Work out the finished part from the listing and answer in its coordinate system (mm). A direction names the side the tool comes from. Give positions to 0.01 mm unless a question says otherwise; leave off trailing zeros. Write each loop counter-clockwise with the first axis right and the second up, starting at its lowest first coordinate (ties: lowest second). Pieces come first, ordered by that corner, then holes. Notation, with made-up numbers: (65.25, -9) -> (112.25, -9) arc R6 cw to (112.25, -3) -> close; hole circle Ø2 at (86.5, 66). An arc over 180 degrees is marked (long way). Use a Markdown table: item, result. Add a question column.
Q1. For a pull along Z with two mould halves and no side action, classify faces 1 (the face through (0, 20, -51)), 2 (the face through (172, 39, -100)), 3 (the face through (180, 60, -93.12)), 4 (the face through (323.197, 20.28, -54.391)) as pulls with the +Z half, pulls with the -Z half, needs draft (parallel to the pull), parting line crosses it, or undercut.
Q2. Each of these flat-tipped pins is pushed along its axis until it touches: pin 1 Ø12 at (x, z) = (263, -63.5) entering from +Y; pin 2 Ø2 at (y, z) = (52.5, -96.5) entering from -X; pin 3 Ø5 at (x, y) = (210.5, 40) entering from +Z; pin 4 Ø0.5 at (x, y) = (339, 64) entering from +Z. Where does it stop, or does it pass through?
Q3. Section D-D, the plane z = -59.5 is taken. Give the vertices of the cut face in (x, y), plus the area to 3 significant figures.
Q4. Consider line 1 (X direction, y = 5, z = -65.5); line 2 (X direction, y = 13.5, z = -64.5); line 3 (Y direction, x = 285.5, z = -70). Determine where each line is inside the solid, lowest interval first.
Q5. For faces 5 (the face through (33.144, 60, -97)), 6 (the face through (340, 22, -49)), 7 (the face through (331.968, 60, -46)), 8 (the face through (231, 80, -95)), 9 (the face through (338.282, 60, -47)), determine the directions among +Z, -Z, +X, -X, +Y, -Y from which every point of the face is accessible in a straight line to the end or side of a thin tool.
Q6. Section B-B, the plane x = 82.5 is taken. Give the vertices of the cut face in (y, z).
Q7. Section A-A, the plane z = -12 is taken. Give the vertices of the cut face in (x, y), plus the area to 3 significant figures.
Q8. Section C-C, the plane y = 51 is taken. Give the vertices of the cut face in (x, z).
Autodesk Inventor part; units mm, degrees
ref_plane "YZ Plane" through (0, 0, 0) normal (1, 0, 0) x (0, 1, 0)
ref_plane "XZ Plane" through (0, 0, 0) normal (0, 1, 0) x (-1, 0, 0)
ref_plane "XY Plane" through (0, 0, 0) normal (0, 0, 1) x (1, 0, 0)
sketch "Sketch1" plane through (0, 0, 0) normal (0, 1, 0) x (-1, 0, 0)
  line L0 (0, 0) -> (-340, 0)
  line L1 (-340, 0) -> (-340, -100)
  line L2 (-340, -100) -> (0, -100)
  line L3 (0, -100) -> (0, 0)
  dimension "d0" = 340
  dimension "d1" = 100
extrude "Extrusion1" add sketch "Sketch1" along normal blind 40
sketch "Sketch2" plane through (0, 40, 0) normal (0, 1, 0) x (1, 0, 0)
  circle A0 centre (302.5068, 47.875) radius 21.6916
  circle A1 centre (202.5481, 47.875) radius 21.6916
  circle A2 centre (96.2761, 47.875) radius 21.6916
  circle A3 centre (302.5068, 47.875) radius 21.6916
  point P0 (0, 0)
extrude "Extrusion2" cut sketch "Sketch2" against normal blind 500
sketch "Sketch3" plane through (0, 40, 0) normal (0, 1, 0) x (1, 0, 0)
  line L0 (340, 100) -> (0, 100)
  line L1 (33.1442, 93.1195) -> (340, 93.1195)
  line L2 (340, 93.1195) -> (340, 100)
  line L3 (340, 100) -> (33.1442, 100)
  line L4 (33.1442, 100) -> (33.1442, 93.1195)
  point P0 (0, 0)
extrude "Extrusion3" add sketch "Sketch3" along normal blind 40
sketch "Sketch4" plane through (0, 40, 0) normal (0, 1, 0) x (1, 0, 0)
  line L0 (340, 93.1195) -> (33.1442, 93.1195)
  line L1 (338.2816, 0) -> (331.9684, 0)
  line L2 (331.9684, 0) -> (331.9684, 93.1195)
  line L3 (331.9684, 93.1195) -> (338.2816, 93.1195)
  line L4 (338.2816, 93.1195) -> (338.2816, 0)
  point P0 (0, 0)
extrude "Extrusion4" add sketch "Sketch4" along normal blind 40
Result set:
| question | item | result |
|---|---|---|
| 1 | face 1 | needs draft |
| 1 | face 2 | pulls with the -Z half |
| 1 | face 3 | pulls with the +Z half |
| 1 | face 4 | undercut |
| 2 | pin 1 | stops at y = 40 |
| 2 | pin 2 | stops at x = 33.14 |
| 2 | pin 3 | stops at z = 0 |
| 2 | pin 4 | stops at z = -93.12 |
| 3 | outline | (0, 0) -> (77.96, 0) -> (77.96, 40) -> (0, 40) -> close; (114.59, 0) -> (184.23, 0) -> (184.23, 40) -> (114.59, 40) -> close; (220.86, 0) -> (284.19, 0) -> (284.19, 40) -> (220.86, 40) -> close; (320.82, 0) -> (340, 0) -> (340, 40) -> (338.28, 40) -> (338.28, 80) -> (331.97, 80) -> (331.97, 40) -> (320.82, 40) -> close |
| 3 | area | 9,460 mm2 |
| 4 | line 1 | x = 0 to 83.63, 108.92 to 189.9, 215.19 to 289.86, 315.15 to 340 |
| 4 | line 2 | x = 0 to 82.34, 110.21 to 188.61, 216.48 to 288.57, 316.44 to 340 |
| 4 | line 3 | y = 0 to 40 |
| 5 | face 5 | +Z, -Z, -X, +Y |
| 5 | face 6 | +Z, -Z, +X, +Y, -Y |
| 5 | face 7 | +Z, -X, +Y |
| 5 | face 8 | +Z, -Z, +X, -X, +Y |
| 5 | face 9 | +Z, +X, +Y |
| 6 | outline | (0, -100) -> (80, -100) -> (80, -93.12) -> (40, -93.12) -> (40, -64.63) -> (0, -64.63) -> close; (0, -31.12) -> (40, -31.12) -> (40, 0) -> (0, 0) -> close |
| 7 | outline | (0, 0) -> (340, 0) -> (340, 40) -> (338.28, 40) -> (338.28, 80) -> (331.97, 80) -> (331.97, 40) -> (0, 40) -> close |
| 7 | area | 13,900 mm2 |
| 8 | outline | (33.14, -100) -> (340, -100) -> (340, -93.12) -> (338.28, -93.12) -> (338.28, 0) -> (331.97, 0) -> (331.97, -93.12) -> (33.14, -93.12) -> close |
